Read the model definition and answer for the solid it produces. Units are mm, in the model's axes. A direction names the side the tool comes from. Give positions to 0.01 mm unless a question says otherwise; leave off trailing zeros. Write each loop counter-clockwise with the first axis right and the second up, starting at its lowest first coordinate (ties: lowest second). Pieces come first, ordered by that corner, then holes. Notation, with made-up numbers: (59.25, 47.5) -> (118.25, 47.5) arc R15 ccw to (118.25, 66.5) -> close; hole circle Ø5 at (68.25, 30.25). An arc over 180 degrees is marked (long way). Write item = value, one per line.
from build123d import *

# Parameters (mm, degrees)
SKETCH1_R          = 53.34
EXTRUDE1_DEPTH     = 54.61
FILLET1_R          = 5
SKETCH2_R          = 27.432
CUT_EXTRUDE1_DEPTH = 17.78
FILLET2_R          = 2
SKETCH3_R          = 34.29
CUT_EXTRUDE2_DEPTH = 10.16
CUT_EXTRUDE2_DRAFT = -70
FILLET3_R          = 35
SKETCH4_R          = 6.375629418
CUT_EXTRUDE3_DEPTH = 15.24
FILLET4_R          = 3


with BuildPart() as part:
    # Sketch1 → Extrude1 (new body)
    with BuildSketch(Plane.XY):
        Circle(SKETCH1_R)
    extrude(amount=EXTRUDE1_DEPTH)

    # Fillet1
    fillet1_edges = [part.edges().sort_by_distance(p)[0] for p in [
        (-53.34, 0, 0),
        (-53.34, 0, 54.61),
    ]]
    fillet(fillet1_edges, radius=FILLET1_R)

    # Sketch2 → Cut-Extrude1 (cut)
    with BuildSketch(Plane(origin=(0, 0, 0), x_dir=(-1, 0, 0), z_dir=(0, 0, -1))):
        Circle(SKETCH2_R)
    extrude(amount=-CUT_EXTRUDE1_DEPTH, mode=Mode.SUBTRACT)

    # Fillet2
    fillet2_edges = [part.edges().sort_by_distance(p)[0] for p in [
        (27.432, 0, 0),
    ]]
    fillet(fillet2_edges, radius=FILLET2_R)


with BuildPart() as cut_extrude2_tool:
    # Sketch3 → Cut-Extrude2 (with draft: the straight prism first)
    with BuildSketch(Plane.XY.offset(54.61)):
        Circle(SKETCH3_R)
    extrude(amount=-CUT_EXTRUDE2_DEPTH)
    # Cut-Extrude2: the draft: its side faces are tilted about the plane it starts from
    cut_extrude2_sides = [cut_extrude2_tool.faces().sort_by_distance(p)[0] for p in [
        (-34.29, 0, 49.53),
    ]]
    draft(cut_extrude2_sides, Plane.XY.offset(54.61), CUT_EXTRUDE2_DRAFT)


with BuildPart() as part_1:
    add(part.part)

    # Cut-Extrude2: cut by cut_extrude2_tool
    add(cut_extrude2_tool.part, mode=Mode.SUBTRACT)

    # Fillet3
    fillet3_edges = [part_1.edges().sort_by_distance(p)[0] for p in [
        (-34.29, 0, 54.61),
    ]]
    fillet(fillet3_edges, radius=FILLET3_R)

    # Sketch4 → Cut-Extrude3 (cut)
    with BuildSketch(Plane.XY.offset(44.45)):
        Circle(SKETCH4_R)
    extrude(amount=-CUT_EXTRUDE3_DEPTH, mode=Mode.SUBTRACT)

    # Fillet4
    fillet4_edges = [part_1.edges().sort_by_distance(p)[0] for p in [
        (-6.375629418, 0, 44.45),
    ]]
    fillet(fillet4_edges, radius=FILLET4_R)


solid = part_1.part
(1) Given P1, Ø6, axis at y = 28.5, z = 48, coming from the +X side; P2, Ø5, axis at x = -2, y = 27.5, coming from the +Z side; P3, Ø5, axis at y = 8.5, z = 37.5, coming from the -X side; P4, Ø3, axis at x = 25, y = -26.5, coming from the -Z side, each flat-ended and moving along its own axis, determine where each tip first touches the part or whether it passes through.
Checks:
P1 = 46.85
P2 = 53.03
P3 = -53
P4 = 0
(2) A tool of negligible diameter and unlimited length cuts with its end or side. For faces 1 (the flat face through (0, 0, 29.21)), 2 (the flat face through (-11, -39.2, 54.61)), 3 (the cylindrical face through (5.95, -26.78, 9.78)), from which of +Z, -Z, +X, -X, +Y, -Y can it reach the whole face along a straight path? Write none if from no direction.
Checks:
face_1 = +Z
face_2 = +Z, +X, -X, +Y, -Y
face_3 = -Z
(3) For a pull along X with two mould halves and no side action, classify faces 4 (the flat face through (0, 0, 17.78)), 5 (the flat face through (21, 22, 0)), 6 (the cylindrical face through (-6.944, 52.886, 26.993)) as released by +X, released by -X, zero draft, split by the parting line, or undercut.
Checks:
face_4 = undercut
face_5 = zero draft
face_6 = split by the parting line
(4) Consider L1, parallel to Y at x = 0, z = 9; L2, parallel to Y at x = 0, z = 35.5; L3, parallel to Y at x = 1, z = 20.5. Determine where each line is inside the solid, lowest interval first.
Checks:
L1 = -53.34 to -27.43, 27.43 to 53.34
L2 = -53.34 to -6.38, 6.38 to 53.34
L3 = -53.33 to 53.33
(5) The part is cut by section A-A on z = 15.5. Determine the outline of the cut face in (x, y).
Checks:
outline = circle Ø106.68 at (0, 0); hole circle Ø54.86 at (0, 0)
(6) The part is cut by section B-B on z = 22. Determine the outline of the cut face in (x, y).
Checks:
outline = circle Ø106.68 at (0, 0)
